The model under review builds one solid part; all positions refer to its coordinate system, in mm. Face numbers are marked on the shaded views. A direction names the side the tool comes from. Round coordinates to 2 decimals unless told otherwise and drop trailing zeros. Loops run counter-clockwise (first coordinate to the right, second up) from the corner with the lowest first, then second, coordinate; pieces in that order, holes last. Notation, with made-up numbers: (13.5, -34) -> (26.5, -34) arc R11 ccw to (26.5, -25) -> close; hole circle Ø5 at (25.5, 60). An arc over 180 degrees is marked (long way). Use CSV: the item, a comma, the result in double quotes. Start each with the question number.
Autodesk Inventor part; units mm, degrees
ref_plane "YZ Plane" through (0, 0, 0) normal (1, 0, 0) x (0, 1, 0)
ref_plane "XZ Plane" through (0, 0, 0) normal (0, 1, 0) x (-1, 0, 0)
ref_plane "XY Plane" through (0, 0, 0) normal (0, 0, 1) x (1, 0, 0)
sketch "スケッチ1" plane through (0, 0, 0) normal (0, 1, 0) x (-1, 0, 0)
  line L0 (3, 26.15) -> (-3, 26.15)
  line L1 (-3, 26.15) -> (-3, -21.5)
  line L2 (-3, -21.5) -> (3, -21.5)
  line L3 (3, -21.5) -> (3, 26.15)
  line L4 (4.2, 0) -> (-4.2, 0) construction
  line L5 (4.2, 9) -> (-4.2, 9) construction
  line L6 (4.2, -9) -> (-4.2, -9) construction
  line L7 (0, -31.03) -> (0, 35.68) construction
  circle A0 centre (0, 9) radius 2
  circle A1 centre (0, -9) radius 2
  line L8 (0, 26.15) -> (0, -21.5) construction
  line L9 (3, 20.15) -> (-3, 20.15)
  line L10 (3, -15.5) -> (-3, -15.5)
  line L11 (3, 26.15) -> (-3, 20.15) construction
  line L12 (3, -15.5) -> (-3, -21.5) construction
  circle A2 centre (0, 23.15) radius 1.25
  circle A3 centre (0, -18.5) radius 1.25
  line L13 (-3, 18.15) -> (3, 18.15)
  line L14 (-3, -13.5) -> (3, -13.5)
  point P0 (0, 0)
  dimension "d0" = 6
  dimension "d1" = 9
  dimension "d2" = 9
  dimension "d3" = 4
  dimension "d4" = 12.5
  dimension "d5" = 17.15
  dimension "d6" = 6
  dimension "d7" = 6
  dimension "d8" = 2.5
  dimension "d11" = 4.5
  dimension "d12" = 9.15
extrude "押し出し1" add sketch "スケッチ1" along normal blind 2 contours L3 L13 L1 L9 | L3 L14 L1 L13 | L3 L10 L1 L14 | A0 | A1
extrude "押し出し2" add sketch "スケッチ1" against normal blind 8 contours L3 L13 L1 L9 | L3 L10 L1 L14
extrude "押し出し3" add sketch "スケッチ1" along normal blind 3 from surface at -8 contours L3 L9 L1 L0 | L3 L2 L1 L10
extrude "押し出し4" add sketch "スケッチ1" against normal blind 2.8 contours A0 | A1
chamfer "面取り1" distance 0.3 angle 45 2 edges at (2, -2.8, 9) (2, -2.8, -9)
properties part number "housing_xl320"
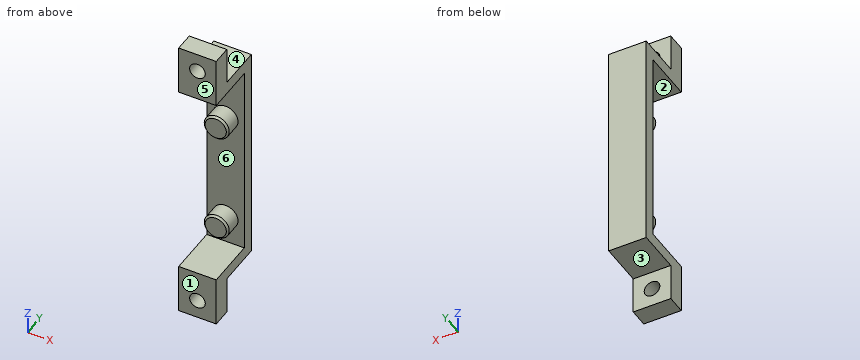
1. For the marked faces 1 and 2, list the 3-axis set-ups (+Z, -Z, +X, -X, +Y, -Y) from which the entire face can be reached by the end or side of a thin tool; tool diameter is ignored.
2. Take a section at D-D, the plane x = -2.55. Give the boundary of the cut face in (y, z).
3. Take a section at C-C, the plane z = 9. Give the boundary of the cut face in (x, y), then the cut area to 3 significant figures.
4. For line 1 along Z through (x, y) = (0, -7.2); line 2 along Z through (x, y) = (-2.5, -1.25); line 3 along Z through (x, y) = (2, -5.25), list the stretches that pass through material, from the lowest coordinate up. Write a range as from..to.
5. The part is to be moulded in two halves that separate along Z. For the marked faces 3, 4, 5 and 6, say which applies: pulls with the +Z half, pulls with the -Z half, needs draft (parallel to the pull), parting line crosses it, or undercut.
6. Take a section at B-B, the plane z = 23.15. Give the boundary of the cut face in (x, y), then the cut area to 3 significant figures.
7. Take a section at A-A, the plane y = -1.75. Give the boundary of the cut face in (x, z), then the cut area to 3 significant figures.
8. Clearance check with flat-ended pins moving along their axes: P1, Ø6, axis at y = -4, z = 7, coming from the +X side; P2, Ø3, axis at x = 0.5, y = -3, coming from the +Z side; P3, Ø1.7, axis at x = -0.5, z = 9, coming from the -Y side. State where each tip first meets the part, or that it passes through.
Results:
1,face 1,"+Z, -Z, +X, -X, -Y"
1,face 2,"+X, -X, -Y"
2,outline,"(-8, -21.5) -> (-5, -21.5) -> (-5, -15.5) -> (2, -15.5) -> (2, 20.15) -> (-5, 20.15) -> (-5, 26.15) -> (-8, 26.15) -> (-8, 18.15) -> (0, 18.15) -> (0, -13.5) -> (-8, -13.5) -> close"
3,outline,"(-3, 0) -> (-2, 0) -> (-2, -2.5) -> (-1.7, -2.8) -> (1.7, -2.8) -> (2, -2.5) -> (2, 0) -> (3, 0) -> (3, 2) -> (-3, 2) -> close"
3,area,"23.1 mm²"
4,line 1,"-21.5..-19.75, -17.25..-13.5, 18.15..21.9, 24.4..26.15"
4,line 2,"-15.5..-13.5, 18.15..20.15"
4,line 3,"-21.5..-13.5, 18.15..26.15"
5,face 3,"pulls with the -Z half"
5,face 4,"pulls with the +Z half"
5,face 5,"needs draft"
5,face 6,"undercut"
6,outline,"(-3, -8) -> (-1.25, -8) -> (-1.25, -5) -> (-3, -5) -> close; (1.25, -8) -> (3, -8) -> (3, -5) -> (1.25, -5) -> close"
6,area,"10.5 mm²"
7,outline,"(-3, -15.5) -> (3, -15.5) -> (3, -13.5) -> (-3, -13.5) -> close; (-3, 18.15) -> (3, 18.15) -> (3, 20.15) -> (-3, 20.15) -> close; circle Ø4 at (0, -9); circle Ø4 at (0, 9)"
7,area,"49.1 mm²"
8,P1,"x = 2"
8,P2,"z = 20.15"
8,P3,"y = -2.8"
